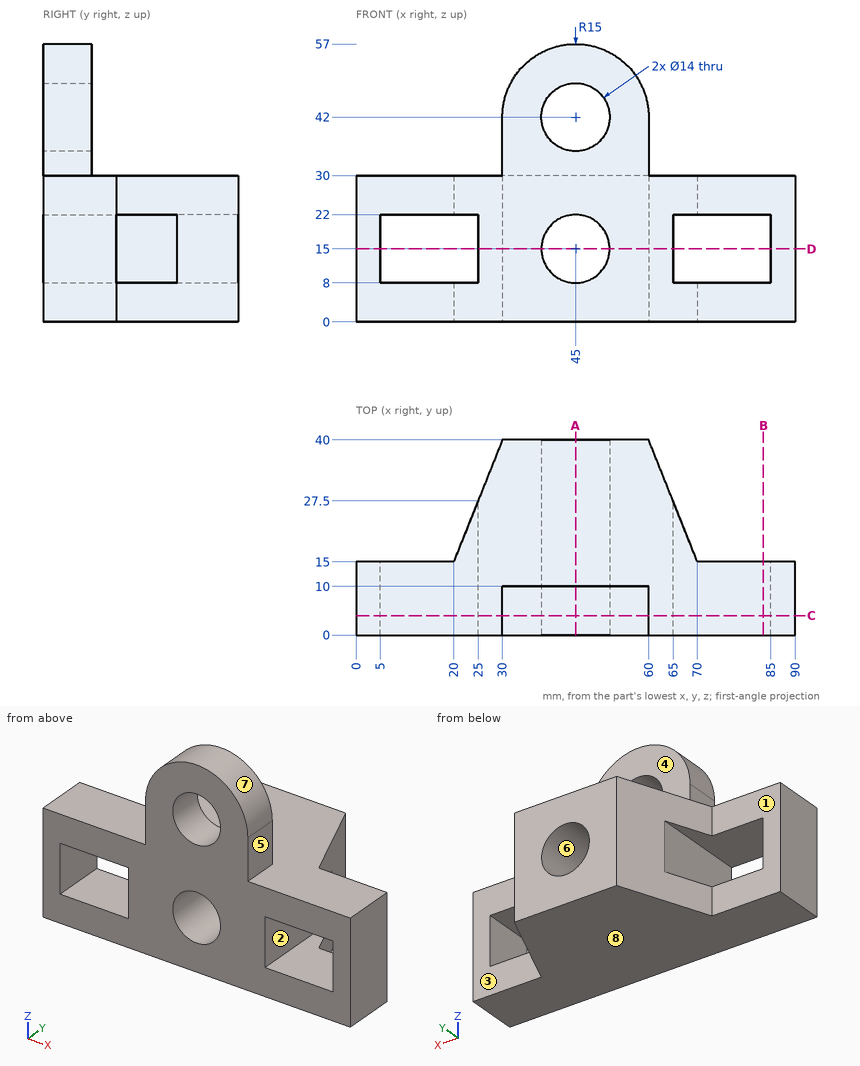
Drawing for the job (mm, zero at the part's lowest x, y, z). A direction names the side the tool comes from. Round coordinates to 2 decimals unless told otherwise and drop trailing zeros. Write each loop counter-clockwise with the first axis right and the second up, starting at its lowest first coordinate (ties: lowest second). Pieces come first, ordered by that corner, then holes. Notation, with made-up numbers: M 73.5,21.5 L 112.5,21.5 A30 ccw 112.5,54.5 Z; hole C 80,56 d9. An arc over 180 degrees is marked long. Answer as a JSON object with one key per item and string values. Group by question number.
(1) Drill centre lines: L1, parallel to X at y = 3, z = 42; L2, parallel to Y at x = 34, z = 46; L3, parallel to Z at x = 55, y = 24. Where is each one in solid material? Low to high.
(2) Mould opens along X. For the marked faces 5, 6, 7 and 8 say: pulls with the +X half, pulls with the -X half, needs draft (parallel to the pull), parting line crosses it, or undercut.
(3) Which spindle directions (+Z, -Z, +X, -X, +Y, -Y) get a long thin tool onto all of the face, cutting with end or side? Do the marked faces 1, 2, 3 and 4. Say none if no direction does.
(4) Flat gauge pins, fed straight in: pin 1 (22 mm diameter, centred on x = 7, z = 13, fed in from +Y); pin 2 (1 mm diameter, centred on x = 45.5, y = 10.5, fed in from -Z); pin 3 (8 mm diameter, centred on x = 48, z = 44.5, fed in from +Y); pin 4 (5 mm diameter, centred on y = 7.5, z = 34, fed in from -X). Where does each tip first touch, or does it go through?
(5) Cut at D-D (z = 15). Give the cut face in (x, y), and give its area (3 significant figures).
(6) Cut at A-A (x = 45). Give the cut face in (y, z).
(7) Cut at B-B (x = 83.5). Give the cut face in (y, z), and give its area (3 significant figures).
(8) Cut at C-C (y = 4). Give the cut face in (x, z).
Responses:
{
 "1": {"L1": "x = 30 to 38, 52 to 60", "L2": "y = 0 to 10", "L3": "z = 0 to 30"},
 "2": {"face 5": "pulls with the +X half", "face 6": "undercut", "face 7": "parting line crosses it", "face 8": "needs draft"},
 "3": {"face 1": "+Z, -Z, -X, +Y", "face 2": "+Y, -Y", "face 3": "+Z, -Z, +X, +Y", "face 4": "+Z, +X, -X, +Y"},
 "4": {"pin 1": "stops at y = 15", "pin 2": "stops at z = 0", "pin 3": "stops at y = 10", "pin 4": "stops at x = 30"},
 "5": {"outline": "M 0,0 L 5,0 L 5,15 L 0,15 Z; M 25,0 L 38,0 L 38,40 L 30,40 L 25,27.5 Z; M 52,0 L 65,0 L 65,27.5 L 60,40 L 52,40 Z; M 85,0 L 90,0 L 90,15 L 85,15 Z", "area": "1,130 mm2"},
 "6": {"outline": "M 0,0 L 40,0 L 40,8 L 0,8 Z; M 0,22 L 40,22 L 40,30 L 10,30 L 10,35 L 0,35 Z; M 0,49 L 10,49 L 10,57 L 0,57 Z"},
 "7": {"outline": "M 0,0 L 15,0 L 15,8 L 0,8 Z; M 0,22 L 15,22 L 15,30 L 0,30 Z", "area": "240 mm2"},
 "8": {"outline": "M 0,0 L 90,0 L 90,30 L 60,30 L 60,42 A15 ccw 30,42 L 30,30 L 0,30 Z; hole M 5,8 L 25,8 L 25,22 L 5,22 Z; hole C 45,15 d14; hole C 45,42 d14; hole M 65,8 L 85,8 L 85,22 L 65,22 Z"}
}
